Read the model definition and answer for the solid it produces. Units are mm, in the model's axes. Round coordinates to 2 decimals unless told otherwise and drop trailing zeros. Loops run counter-clockwise (first coordinate to the right, second up) from the corner with the lowest first, then second, coordinate; pieces in that order, holes last. Notation, with made-up numbers: (27.5, 27.5) -> (83.5, 27.5) arc R23 ccw to (83.5, 38.5) -> close; hole circle Ø9 at (-35, 11.5). An arc over 180 degrees is marked (long way). Put each result on its own line as item: value.
from build123d import *

# Parameters (mm, degrees)
SKETCH_1_W          = 25
SKETCH_1_H          = 80
EXTRUDE_1_DEPTH     = 5
SKETCH_2_R          = 2
CUT_EXTRUDE_1_DEPTH = 6


with BuildPart() as part:
    # 草图1 → 凸台-拉伸1 (new body)
    with BuildSketch(Plane.XY):
        Rectangle(SKETCH_1_W, SKETCH_1_H)
    extrude(amount=-EXTRUDE_1_DEPTH)

    # 草图2 → 切除-拉伸1 (cut, through all)
    with BuildSketch(Plane.XY):
        with Locations((0, 33)):
            Circle(SKETCH_2_R)
        with Locations((0, 23)):
            Circle(SKETCH_2_R)
        with Locations((-5, -34)):
            Circle(SKETCH_2_R)
        with Locations((5, -34)):
            Circle(SKETCH_2_R)
    extrude(amount=-CUT_EXTRUDE_1_DEPTH, mode=Mode.SUBTRACT)


solid = part.part
Item 1: The part is cut by section A-A (x = 0). Determine the outline of the cut face in (y, z), then the cut area to 3 significant figures.
Derived:
outline: (-40, -5) -> (21, -5) -> (21, 0) -> (-40, 0) -> close; (25, -5) -> (31, -5) -> (31, 0) -> (25, 0) -> close; (35, -5) -> (40, -5) -> (40, 0) -> (35, 0) -> close
area: 360 mm^2
Item 2: The part is cut by section B-B (y = -34). Determine the outline of the cut face in (x, z).
Derived:
outline: (-12.5, -5) -> (-7, -5) -> (-7, 0) -> (-12.5, 0) -> close; (-3, -5) -> (3, -5) -> (3, 0) -> (-3, 0) -> close; (7, -5) -> (12.5, -5) -> (12.5, 0) -> (7, 0) -> close
Item 3: The part is cut by section D-D (z = -1.6). Determine the outline of the cut face in (x, y), then the cut area to 3 significant figures.
Derived:
outline: (-12.5, -40) -> (12.5, -40) -> (12.5, 40) -> (-12.5, 40) -> close; hole circle Ø4 at (-5, -34); hole circle Ø4 at (0, 23); hole circle Ø4 at (0, 33); hole circle Ø4 at (5, -34)
area: 1,950 mm^2
Item 4: Find the intervals of material crossed by line 1 along Y through (x, z) = (0, -1.25); line 2 along Y through (x, z) = (-5, -1.65); line 3 along Y through (x, z) = (1.5, -3.25), in increasing order.
Derived:
line 1: y = -40 to 21, 25 to 31, 35 to 40
line 2: y = -40 to -36, -32 to 40
line 3: y = -40 to 21.68, 24.32 to 31.68, 34.32 to 40
Item 5: The part is cut by section C-C (x = -5). Determine the outline of the cut face in (y, z), then the cut area to 3 significant figures.
Derived:
outline: (-40, -5) -> (-36, -5) -> (-36, 0) -> (-40, 0) -> close; (-32, -5) -> (40, -5) -> (40, 0) -> (-32, 0) -> close
area: 380 mm^2
Item 6: Flat-ended cylindrical pins translate along their axes: pin 1 Ø3.5 at (x, y) = (5, -34) entering from +Z; pin 2 Ø6.5 at (x, y) = (0, 33) entering from +Z. Find the tip coordinate at first contact, or state that the pin passes through.
Derived:
pin 1: passes through
pin 2: stops at z = 0
Item 7: For a pull along X with two mould halves and no side action, classify faces 1 (the flat face through (-12.5, -1, -2)), 2 (the cylindrical face through (0, 31, -2)), 3 (the flat face through (0, 40, -2)) as pulls with the +X half, pulls with the -X half, needs draft (parallel to the pull), parting line crosses it, or undercut.
Derived:
face 1: pulls with the -X half
face 2: undercut
face 3: needs draft
